```python
from build123d import *

# Parameters (mm, degrees)
SKETCH_1_W          = 53
SKETCH_1_H          = 53
EXTRUDE_1_DEPTH     = 1
SKETCH_2_W          = 6
SKETCH_2_H          = 6
EXTRUDE_2_DEPTH     = 2.5
SKETCH_3_R          = 2.75
EXTRUDE_3_DEPTH     = 1
SKETCH_4_W          = 6
SKETCH_4_H          = 6
EXTRUDE_4_DEPTH     = 6
SKETCH_5_R          = 2.5
EXTRUDE_5_DEPTH     = 3
SKETCH_6_R          = 3.75
EXTRUDE_6_DEPTH     = 2
EXTRUDE_7_DEPTH     = 6
SKETCH_8_R          = 3
EXTRUDE_8_DEPTH     = 1
SKETCH_9_W          = 6
SKETCH_9_H          = 6
EXTRUDE_9_DEPTH     = 6.5
SKETCH_11_R         = 1.5
CUT_EXTRUDE_1_DEPTH = 52.559407483
FILLET_1_R          = 3


with BuildPart() as part:
    # 草图1 → 凸台-拉伸1 (new body)
    with BuildSketch(Plane(origin=(0, 0, 0), x_dir=(1, 0, 0), z_dir=(0, 1, 0))):
        Rectangle(SKETCH_1_W, SKETCH_1_H)
    extrude(amount=EXTRUDE_1_DEPTH)

    # 草图2 → 凸台-拉伸2 (add)
    with BuildSketch(Plane(origin=(0, 1, 0), x_dir=(1, 0, 0), z_dir=(0, 1, 0))):
        with Locations((-21.5, 15)):
            Rectangle(SKETCH_2_W, SKETCH_2_H)
    extrude(amount=EXTRUDE_2_DEPTH)

    # 草图3 → 凸台-拉伸3 (add)
    with BuildSketch(Plane(origin=(0, 3.5, 0), x_dir=(1, 0, 0), z_dir=(0, 1, 0))):
        with Locations(Location((-21.5, 15, 0), (0, 0, 270))):
            Circle(SKETCH_3_R)
    extrude(amount=EXTRUDE_3_DEPTH)

    # 草图4 → 凸台-拉伸4 (add)
    with BuildSketch(Plane(origin=(0, 4.5, 0), x_dir=(1, 0, 0), z_dir=(0, 1, 0))):
        with Locations((-21.5, 15)):
            Rectangle(SKETCH_4_W, SKETCH_4_H)
    extrude(amount=EXTRUDE_4_DEPTH)

    # 草图5 → 凸台-拉伸5 (add)
    with BuildSketch(Plane.ZY.offset(24.5)):
        with Locations((-15, 7.5)):
            Circle(SKETCH_5_R)
    extrude(amount=EXTRUDE_5_DEPTH)

    # 草图6 → 凸台-拉伸6 (add)
    with BuildSketch(Plane.ZY.offset(27.5)):
        with Locations((-15, 7.5)):
            Circle(SKETCH_6_R)
    extrude(amount=EXTRUDE_6_DEPTH)

    # 草图7 → 凸台-拉伸7 (add)
    with BuildSketch(Plane.ZY.offset(29.5)):
        Polygon((-10.554402927, 7.5), (-12.777201464, 11.35), (-17.222798536, 11.35), (-19.445597073, 7.5), (-17.222798536, 3.65), (-12.777201464, 3.65), align=None)
    extrude(amount=EXTRUDE_7_DEPTH)

    # 草图8 → 凸台-拉伸8 (add)
    with BuildSketch(Plane.ZY.offset(35.5)):
        with Locations((-15, 7.5)):
            Circle(SKETCH_8_R)
    extrude(amount=EXTRUDE_8_DEPTH)

    # 草图9 → 凸台-拉伸9 (add)
    with BuildSketch(Plane.ZY.offset(36.5)):
        with Locations((-15, 7.5)):
            Rectangle(SKETCH_9_W, SKETCH_9_H)
    extrude(amount=EXTRUDE_9_DEPTH)

    # 草图11 → 切除-拉伸1 (cut, through all)
    with BuildSketch(Plane(origin=(0, 1, 0), x_dir=(1, 0, 0), z_dir=(0, 1, 0))):
        with Locations(Location((-23, -23, 0), (0, 0, 270))):
            Circle(SKETCH_11_R)
        with Locations(Location((-23, 23, 0), (0, 0, 270))):
            Circle(SKETCH_11_R)
        with Locations(Location((23, 23, 0), (0, 0, 270))):
            Circle(SKETCH_11_R)
        with Locations(Location((23, -23, 0), (0, 0, 270))):
            Circle(SKETCH_11_R)
    extrude(amount=-CUT_EXTRUDE_1_DEPTH, mode=Mode.SUBTRACT)

    # 圆角1
    fillet_1_edges = [part.edges().sort_by_distance(p)[0] for p in [
        (26.5, 0.5, 26.5),
        (-26.5, 0.5, 26.5),
        (-26.5, 0.5, -26.5),
        (26.5, 0.5, -26.5),
    ]]
    fillet(fillet_1_edges, radius=FILLET_1_R)


solid = part.part
```
Verification items for the finished model (mm, model axes). A direction names the side the tool comes from. Coordinates: 2 decimals unless noted, no trailing zeros. Loops run counter-clockwise (first coordinate to the right, second up) from the corner with the lowest first, then second, coordinate; pieces in that order, holes last. Notation, with made-up numbers: (-8, 46) - (44, 46) arc R37 cw to (44, 85) - close; hole circle Ø6 at (44, -21.5). An arc over 180 degrees is marked (long way). Put each result on its own line as item: value.
Item 1: Draft check along X on faces 1 (the face through (-32, 3.65, -15)), 2 (the face through (-35.5, 4, -15)), 3 (the face through (-36.5, 5, -17)), 4 (the face through (-24.5, 2, -15)). Enter one of: pulls with the +X half, pulls with the -X half, needs draft (parallel to the pull), parting line crosses it, or undercut.
Conclusion:
face 1: needs draft
face 2: undercut
face 3: undercut
face 4: pulls with the -X half
Item 2: Set-up check for faces 5 (the face through (-36.5, 5, -13)), 6 (the face through (-22, 10.5, -15)), 7 (the face through (-22, 2, -12)), 8 (the face through (-36.5, 10, -13)), 9 (the face through (-22, 7, -18)): record each of +Z, -Z, +X, -X, +Y, -Y from which the full face is reachable in a straight line by a thin tool's end or side.
Conclusion:
face 5: +Z, -Y
face 6: +Z, -Z, +X, +Y
face 7: +Z, +X, -X, +Y
face 8: +Z, +Y
face 9: -Z, +X, +Y
Item 3: Section check B-B (z = 4.5). Enter the section's corners in (x, y).
Conclusion:
outline: (-26.5, 0) - (26.5, 0) - (26.5, 1) - (-26.5, 1) - close
Item 4: Section check C-C (y = 6.25). Enter the section's corners in (x, z).
Conclusion:
outline: (-43, -18) - (-36.5, -18) - (-36.5, -17.73) - (-35.5, -17.73) - (-35.5, -18.72) - (-29.5, -18.72) - (-29.5, -18.54) - (-27.5, -18.54) - (-27.5, -17.17) - (-24.5, -17.17) - (-24.5, -18) - (-18.5, -18) - (-18.5, -12) - (-24.5, -12) - (-24.5, -12.83) - (-27.5, -12.83) - (-27.5, -11.46) - (-29.5, -11.46) - (-29.5, -11.28) - (-35.5, -11.28) - (-35.5, -12.27) - (-36.5, -12.27) - (-36.5, -12) - (-43, -12) - close
Item 5: Scan lines: line 1 along X through (y, z) = (0.7, -23); line 2 along X through (y, z) = (4.75, -14); line 3 along Y through (x, z) = (6, 2). Record each from-to range of solid material in increasing order.
Conclusion:
line 1: x = -26.5 to -24.5, -21.5 to 21.5, 24.5 to 26.5
line 2: x = -43 to -27.5, -24.5 to -18.5
line 3: y = 0 to 1
Item 6: Gauge pin test, flat ends, axial feed: pin 1 Ø4 at (x, z) = (-23, 23) entering from +Y; pin 2 Ø2.5 at (x, z) = (-23, -23) entering from +Y (3 decimals); pin 3 Ø1.2 at (y, z) = (3, -14) entering from +X; pin 4 Ø3.5 at (x, z) = (-31.5, -16) entering from -Y. Record the tip position at first contact, or that the pin passes through.
Conclusion:
pin 1: stops at y = 1
pin 2: passes through
pin 3: stops at x = -18.5
pin 4: stops at y = 3.65
Item 7: Section check D-D (x = -20). Enter the section's corners in (y, z).
Conclusion:
outline: (0, -26.5) - (1, -26.5) - (1, -18) - (3.5, -18) - (3.5, -17.3) - (4.5, -17.3) - (4.5, -18) - (10.5, -18) - (10.5, -12) - (4.5, -12) - (4.5, -12.7) - (3.5, -12.7) - (3.5, -12) - (1, -12) - (1, 26.5) - (0, 26.5) - close
Item 8: Section check A-A (x = -7). Enter the section's corners in (y, z), then the cut area to 3 significant figures.
Conclusion:
outline: (0, -26.5) - (1, -26.5) - (1, 26.5) - (0, 26.5) - close
area: 53.0 mm2
